Design review of the part shown in the three views and the two pictorial views. Dimensions are in mm from the part's minimum x, y and z. A direction names the side the tool comes from. Give positions to 0.01 mm unless a question says otherwise; leave off trailing zeros. Write each loop counter-clockwise with the first axis right and the second up, starting at its lowest first coordinate (ties: lowest second). Pieces come first, ordered by that corner, then holes. Notation, with made-up numbers: (31.5, 56) -> (60.5, 56) arc R27 cw to (60.5, 94) -> close; hole circle Ø3 at (-14, -26). An arc over 180 degrees is marked (long way). Use CSV: the item, a comma, the result in double quotes.
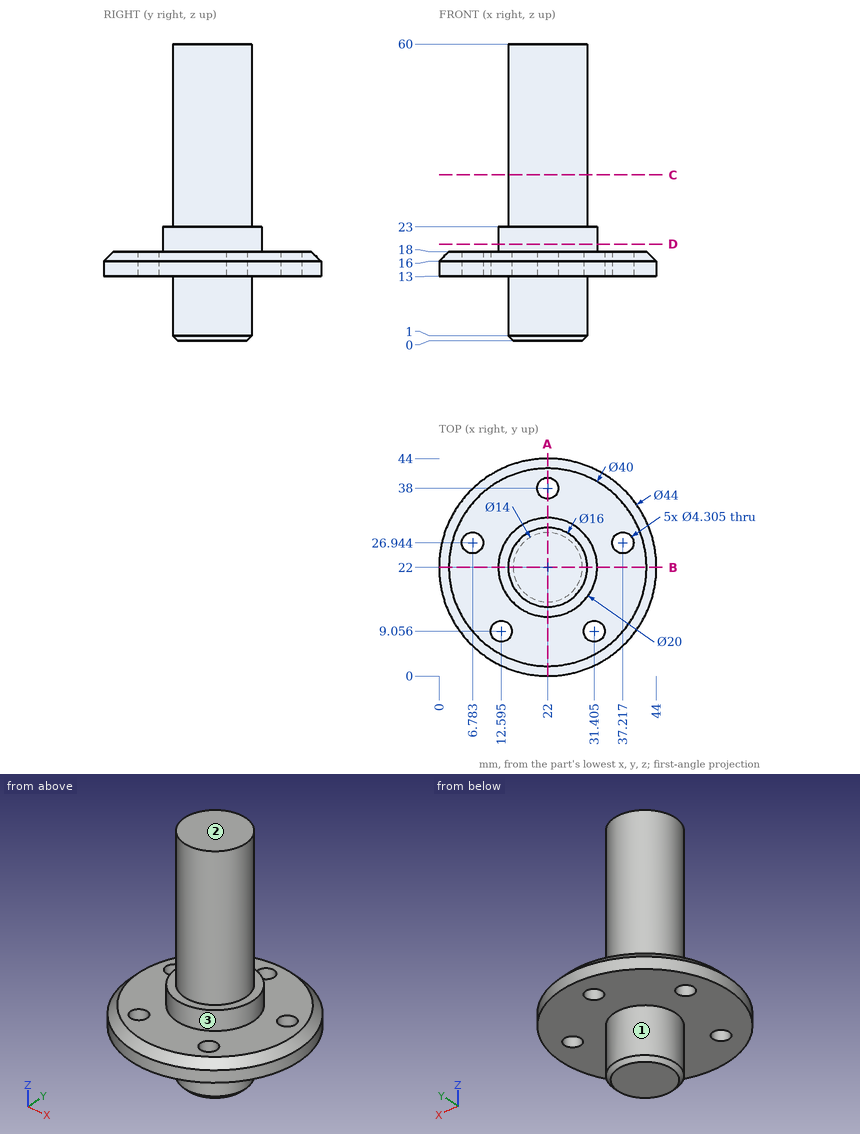
Q1. To check wall thickness, follow probe 1 along Y at (x, z) = (33, 16.5) (1 decimal); probe 2 along Z at (x, y) = (26, 33); probe 3 along Y at (x, z) = (23, 20.5). State the ranges of each line that lie inside material, in increasing order.
Derived:
probe 1,"y = 3.5 to 7.6, 10.5 to 40.5"
probe 2,"z = 13 to 18"
probe 3,"y = 12.05 to 31.95"
Q2. Insertion check: pin 1 (6 mm diameter, centred on x = 28.5, y = 31.5, fed in from -Z); pin 2 (12 mm diameter, centred on y = 17, z = 46, fed in from +X); pin 3 (1 mm diameter, centred on y = 23, z = 42.5, fed in from -X). Each pin has a flat end and moves straight along its axis. Give the tip position at first contact, or say it passes through.
Derived:
pin 1,"stops at z = 13"
pin 2,"stops at x = 30"
pin 3,"stops at x = 14.02"
Q3. Consider section C-C (z = 33.5). Write out the cut boundary in (x, y), then the cut area to 3 significant figures.
Derived:
outline,"circle Ø16 at (22, 22)"
area,"201 mm2"
Q4. Consider section B-B (y = 22). Write out the cut boundary in (x, z), then the cut area to 4 significant figures.
Derived:
outline,"(0, 13) -> (14, 13) -> (14, 1) -> (15, 0) -> (29, 0) -> (30, 1) -> (30, 13) -> (44, 13) -> (44, 16) -> (42, 18) -> (32, 18) -> (32, 23) -> (30, 23) -> (30, 60) -> (14, 60) -> (14, 23) -> (12, 23) -> (12, 18) -> (2, 18) -> (0, 16) -> close"
area,"1,115 mm2"
Q5. Consider section D-D (z = 19.5). Write out the cut boundary in (x, y).
Derived:
outline,"circle Ø20 at (22, 22)"
Q6. Consider section A-A (x = 22). Write out the cut boundary in (y, z).
Derived:
outline,"(0, 13) -> (14, 13) -> (14, 1) -> (15, 0) -> (29, 0) -> (30, 1) -> (30, 13) -> (35.85, 13) -> (35.85, 18) -> (32, 18) -> (32, 23) -> (30, 23) -> (30, 60) -> (14, 60) -> (14, 23) -> (12, 23) -> (12, 18) -> (2, 18) -> (0, 16) -> close; (40.15, 13) -> (44, 13) -> (44, 16) -> (42, 18) -> (40.15, 18) -> close"
Q7. Machinability: for the marked faces 1, 2 and 3, which of the approach directions +Z, -Z, +X, -X, +Y, -Y give a long, thin tool a straight path to every point of the face, cutting with its end or side? Answer none if there is none.
Derived:
face 1,"-Z"
face 2,"+Z, +X, -X, +Y, -Y"
face 3,"+Z"
